```python
from build123d import *

# Parameters (mm, degrees)
BOSS_EXTRUDE1_START = 2.8702
SKETCH3_R           = 2.8702
BOSS_EXTRUDE1_DEPTH = 2.8702
FILLET1_R           = 2.8702
CUT_EXTRUDE1_START  = 2.54
SKETCH4_R           = 1.397
CUT_EXTRUDE1_DEPTH  = 2.54


with BuildPart() as part:
    # Sketch1 → Revolve1 (revolve)
    with BuildSketch(Plane(origin=(0, 0, 0), x_dir=(1, 0, 0), z_dir=(0, 1, 0))):
        Polygon((-36.261655476, 25.478138479), (-30.153813644, 24.589138479), (9.800386356, 24.589138479), (17.401896005, 23.560438479), (53.800096005, 23.560438479), (53.800096005, 20.690238479), (-205.705055476, 20.690238479), (-205.705055476, 26.824338479), (-120.792855476, 26.824338479), (-120.792855476, 25.478138479), align=None)
    revolve(axis=Axis((53.800096005, 0, -20.690238479), (-1, 0, 0)))

    # Sketch3 → Boss-Extrude1 (add)
    with BuildSketch(Plane(origin=(53.800096005, 0, 0), x_dir=(0, 0, -1), z_dir=(1, 0, 0)).offset(BOSS_EXTRUDE1_START)):
        with Locations((20.690238479, 0)):
            Circle(SKETCH3_R)
    extrude(amount=-BOSS_EXTRUDE1_DEPTH)

    # Fillet1
    fillet1_edges = [part.edges().sort_by_distance(p)[0] for p in [
        (56.670296005, 0, -17.820038479),
    ]]
    fillet(fillet1_edges, radius=FILLET1_R)

    # Sketch4 → Cut-Extrude1 (cut)
    with BuildSketch(Plane(origin=(0, 0, 0), x_dir=(1, 0, 0), z_dir=(0, 1, 0)).offset(CUT_EXTRUDE1_START)):
        with Locations((20.272096005, 20.690238479)):
            Circle(SKETCH4_R)
    extrude(amount=CUT_EXTRUDE1_DEPTH, mode=Mode.SUBTRACT)


solid = part.part
```
Can you work these out from the model? Positions are in its coordinate system, mm. A direction names the side the tool comes from. Coordinates: 2 decimals unless noted, no trailing zeros. Loops run counter-clockwise (first coordinate to the right, second up) from the corner with the lowest first, then second, coordinate; pieces in that order, holes last. Notation, with made-up numbers: M 11,-35.75 L 34,-35.75 A37 ccw 34,0.25 Z; hole C 7.5,26.25 d4. An arc over 180 degrees is marked long. Put each result on its own line as item: value. Start each with the question number.
(1) Imagine slicing it at C-C on x = -48. List the corners of the cut face in (y, z) for me, and give its area (3 significant figures).
(2) I need wall thicknesses on probe 1 along Y at (x, z) = (-161, -24.5); probe 2 along X at (y, z) = (4.75, -22.5); probe 3 along Z at (x, y) = (-85.5, -0.5). Which ranges of each line are inside material? Lowest first, please.
(3) We'd pull the mould along Z, two halves only. Please class faces 1 (the face through (-77.936, -0.211, -15.907)), 2 (the face through (-205.705, 0, -21)): +Z half, -Z half, draft (parallel to the pull), parting line (faces both ways), or undercut.
(4) Imagine slicing it at A-A on y = 0. List the corners of the cut face in (x, z) for me, and give its area (3 significant figures).
(5) Will these pins go through, and if not, where does the flat tip stop? pin 1 Ø3 at (x, z) = (-46, -22) entering from -Y; pin 2 Ø1 at (y, z) = (-4, -16.5) entering from +X; pin 3 Ø4 at (x, z) = (13.5, -25) entering from -Y.
(6) Imagine slicing it at B-B on x = 14. List the corners of the cut face in (y, z) for me, and give its area (3 significant figures).
(7) Which directions (+Z, -Z, +X, -X, +Y, -Y) give clear straight access to the entire face, cutting with the end or side of a thin tool? Please do faces 3 (the face through (-162.65, -1.84, -26.54)), 4 (the face through (35.86, -2.55, -22.01)).
Worked answers:
1. outline: C 0,-20.69 d9.58
1. area: 72.0 mm2
2. probe 1: y = -4.81 to 4.81
2. probe 2: x = -205.71 to -120.79
2. probe 3: z = -25.45 to -15.93
3. face 1: parting line
3. face 2: draft
4. outline: M -205.71,-26.82 L -120.79,-26.82 L -120.79,-25.48 L -36.26,-25.48 L -30.15,-24.59 L 9.8,-24.59 L 17.4,-23.56 L 53.8,-23.56 A2.87 ccw 53.8,-17.82 L 17.4,-17.82 L 9.8,-16.79 L -30.15,-16.79 L -36.26,-15.9 L -120.79,-15.9 L -120.79,-14.56 L -205.71,-14.56 Z
4. area: 2,490 mm2
5. pin 1: stops at y = -4.79
5. pin 2: stops at x = -120.79
5. pin 3: stops at y = -2.53
6. outline: C 0,-20.69 d6.66
6. area: 34.8 mm2
7. face 3: +X, -X
7. face 4: +X
